Input: part model. Units: mm. Frame: model coordinates. Face numbers are marked on the shaded views. Round coordinates to 2 decimals unless told otherwise and drop trailing zeros. Loops run counter-clockwise (first coordinate to the right, second up) from the corner with the lowest first, then second, coordinate; pieces in that order, holes last. Notation, with made-up numbers: (70.25, -28) -> (125.25, -28) arc R17 cw to (125.25, -22) -> close; hole circle Ø2 at (-14, 26.25). An arc over 180 degrees is marked (long way). Answer as a JSON object with one key per item and string values.
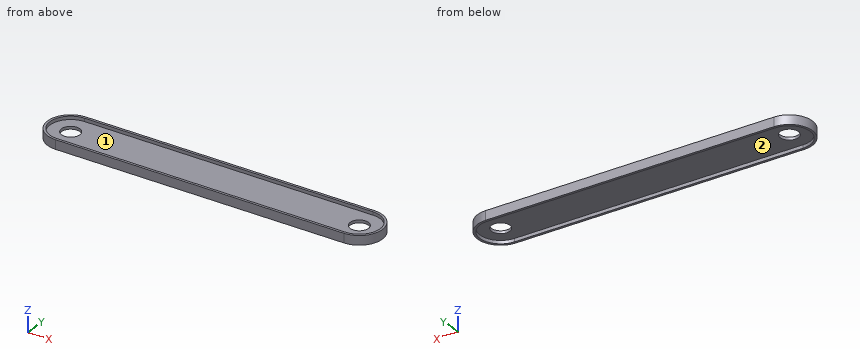
```python
from build123d import *

# Parameters (mm, degrees)
SKETCH1_R           = 20
BOSS_EXTRUDE1_DEPTH = 10
CUT_EXTRUDE1_DEPTH  = 7


with BuildPart() as part:
    # Sketch1 → Boss-Extrude1 (new, symmetric)
    with BuildSketch(Plane.XY):
        with BuildLine():
            Line((-312.5, -50), (312.5, -50))
            ThreePointArc((312.5, -50), (362.5, 0), (312.5, 50))
            Line((312.5, 50), (-312.5, 50))
            ThreePointArc((-312.5, 50), (-362.5, 0), (-312.5, -50))
        make_face()
        with Locations((312.5, 0)):
            Circle(SKETCH1_R, mode=Mode.SUBTRACT)
        with Locations((-312.5, 0)):
            Circle(SKETCH1_R, mode=Mode.SUBTRACT)
    extrude(amount=BOSS_EXTRUDE1_DEPTH, both=True)

    # Sketch2 → Cut-Extrude1 (cut)
    with BuildSketch(Plane(origin=(0, 0, -10), x_dir=(-1, 0, 0), z_dir=(0, 0, -1))):
        with BuildLine():
            Line((312.5, 45), (-312.5, 45))
            ThreePointArc((-312.5, 45), (-357.5, 0), (-312.5, -45))
            Line((-312.5, -45), (312.5, -45))
            ThreePointArc((312.5, -45), (357.5, 0), (312.5, 45))
        make_face()
    cut_extrude1 = extrude(amount=-CUT_EXTRUDE1_DEPTH, mode=Mode.SUBTRACT)

    # Mirror2: Cut-Extrude1 across plane
    add(cut_extrude1.mirror(Plane.XY), mode=Mode.SUBTRACT)


solid = part.part
```
1) Section C-C, the plane z = 6. Output: boundary loops of the cut face in (x, y), plus the area to 3 significant figures.
Output:
{"outline": "(-312.5, -50) -> (312.5, -50) arc R50 ccw to (312.5, 50) -> (-312.5, 50) arc R50 ccw to start; hole (-312.5, -45) -> (312.5, -45) arc R45 ccw to (312.5, 45) -> (-312.5, 45) arc R45 ccw to start", "area": "7,740 mm^2"}
2) Section A-A, the plane y = 0. Output: boundary loops of the cut face in (x, z), plus the area to 3 significant figures.
Output:
{"outline": "(-362.5, -10) -> (-357.5, -10) -> (-357.5, -3) -> (-332.5, -3) -> (-332.5, 3) -> (-357.5, 3) -> (-357.5, 10) -> (-362.5, 10) -> close; (-292.5, -3) -> (292.5, -3) -> (292.5, 3) -> (-292.5, 3) -> close; (332.5, -3) -> (357.5, -3) -> (357.5, -10) -> (362.5, -10) -> (362.5, 10) -> (357.5, 10) -> (357.5, 3) -> (332.5, 3) -> close", "area": "4,010 mm^2"}
3) Draft query along X for the marked faces 1 and 2. Return one class per face: +X half, -X half, draft (parallel to the pull), parting line (faces both ways), or undercut.
Output:
{"face 1": "undercut", "face 2": "undercut"}
4) Section D-D, the plane y = 34. Output: boundary loops of the cut face in (x, z).
Output:
{"outline": "(-349.16, -10) -> (-341.98, -10) -> (-341.98, -3) -> (341.98, -3) -> (341.98, -10) -> (349.16, -10) -> (349.16, 10) -> (341.98, 10) -> (341.98, 3) -> (-341.98, 3) -> (-341.98, 10) -> (-349.16, 10) -> close"}
5) Section B-B, the plane x = 50. Output: boundary loops of the cut face in (y, z), plus the area to 3 significant figures.
Output:
{"outline": "(-50, -10) -> (-45, -10) -> (-45, -3) -> (45, -3) -> (45, -10) -> (50, -10) -> (50, 10) -> (45, 10) -> (45, 3) -> (-45, 3) -> (-45, 10) -> (-50, 10) -> close", "area": "740 mm^2"}
6) Ray query, probe 1 along X at (y, z) = (0, 1); probe 2 along Y at (x, z) = (-312.5, 0.6); probe 3 along Y at (x, z) = (48, 9). Return the intervals inside material, ascending.
Output:
{"probe 1": "x = -362.5 to -332.5, -292.5 to 292.5, 332.5 to 362.5", "probe 2": "y = -50 to -20, 20 to 50", "probe 3": "y = -50 to -45, 45 to 50"}
7) Contact query for flat-ended pins moving along their axis: P1, Ø1.5, axis at x = -10, y = 26, coming from the -Z side; P2, Ø2, axis at y = -24.5, z = -5, coming from the -X side; P3, Ø2, axis at x = 166, y = -40, coming from the +Z side. Output: stop coordinate, or through.
Output:
{"P1": "stops at z = -3", "P2": "stops at x = -356.63", "P3": "stops at z = 3"}
